Model file for the job. Use its own axes, mm. A direction names the side the tool comes from. Coordinates: 2 decimals unless noted, no trailing zeros. Write each loop counter-clockwise with the first axis right and the second up, starting at its lowest first coordinate (ties: lowest second). Pieces come first, ordered by that corner, then holes. Notation, with made-up numbers: (-27, 42) - (7, 42) arc R22 ccw to (7, 74) - close; hole circle Ø7 at (15.25, -40). An arc over 180 degrees is marked (long way). Put each result on its own line as item: value. Start each with the question number.
1. Saw through at B-B, the plane x = 0. Write the cut outline in (y, z) (1 decimal).
2. Drill centre lines: L1, parallel to Z at x = -21, y = -3 (3 decimals); L2, parallel to X at y = 2, z = -3; L3, parallel to X at y = 2, z = -9. Where is each one in solid material? Low to high. Write a range as from..to.
3. Saw through at D-D, the plane y = -2. Give the number of separate pieces and of enclosed holes in the cut face, plus the area to 3 significant figures.
4. Drop flat-ended pins along their axis: P1, Ø1, axis at y = -1, z = -24, coming from the +X side; P2, Ø4, axis at y = 1.5, z = -6, coming from the +X side; P3, Ø8, axis at y = 12, z = -5, coming from the -X side. Give the stop position or say it passes through.
5. Which spindle directions (+Z, -Z, +X, -X, +Y, -Y) get a long thin tool onto all of the face, cutting with end or side? Do faces 1 (the face through (1.27, 0, -24)), 2 (the face through (0, 0, -25.4)), 3 (the face through (0, 0, -22.225)). Say none if no direction does.
6. Saw through at C-C, the plane z = -12.5. Write the cut outline in (x, y) (1 decimal).
7. Pull direction Y, two halves, no side cores. Call faces 4 (the face through (-2.3, -4.4, 0)), 5 (the face through (-1.27, 0, -24)), 6 (the face through (7.559, 5.796, -3.541)): released by +Y, released by -Y, zero draft, split by the parting line, or undercut.
```python
from build123d import *

# Parameters (mm, degrees)
CUT_EXTRUDE1_DEPTH = 26.4
CUT_EXTRUDE2_DEPTH = 22.225
FILLET1_R          = 2.54


with BuildPart() as part:
    # Sketch1 → Revolve1 (revolve)
    with BuildSketch(Plane(origin=(0, 0, 0), x_dir=(1, 0, 0), z_dir=(0, 1, 0))):
        Polygon((0, 0), (-9.525, 0), (-9.525, 9.525), (-25.4, 9.525), (-25.4, 25.4), (0, 25.4), align=None)
    revolve(axis=Axis((0, 0, -87.406759955), (0, 0, 1)))

    # Sketch2 → Cut-Extrude1 (cut, through all)
    with BuildSketch(Plane(origin=(0, 0, -25.4), x_dir=(-1, 0, 0), z_dir=(0, 0, -1))):
        with BuildLine():
            Line((-1.27, -4.590044254), (-1.27, 4.590044254))
            ThreePointArc((-1.27, 4.590044254), (-4.7625, 0), (-1.27, -4.590044254))
        make_face()
        with BuildLine():
            ThreePointArc((4.7625, 0), (3.790104303, 2.883836962), (1.27, 4.590044254))
            Line((1.27, 4.590044254), (1.27, -4.590044254))
            ThreePointArc((1.27, -4.590044254), (3.790104303, -2.883836962), (4.7625, 0))
        make_face()
    extrude(amount=-CUT_EXTRUDE1_DEPTH, mode=Mode.SUBTRACT)

    # Sketch3 → Cut-Extrude2 (cut)
    with BuildSketch(Plane.XY):
        with BuildLine():
            ThreePointArc((1.27, 4.590044254), (0, 4.7625), (-1.27, 4.590044254))
            Line((-1.27, 4.590044254), (-1.27, -4.590044254))
            ThreePointArc((-1.27, -4.590044254), (0, -4.7625), (1.27, -4.590044254))
            Line((1.27, -4.590044254), (1.27, 4.590044254))
        make_face()
    extrude(amount=-CUT_EXTRUDE2_DEPTH, mode=Mode.SUBTRACT)

    # Fillet1
    fillet1_edges = [part.edges().sort_by_distance(p)[0] for p in [
        (9.525, 0, -9.525),
    ]]
    fillet(fillet1_edges, radius=FILLET1_R)


solid = part.part
```
Final values:
1. outline: (-25.4, -25.4) - (25.4, -25.4) - (25.4, -9.5) - (12.1, -9.5) arc R2.5 cw to (9.5, -7) - (9.5, 0) - (4.8, 0) - (4.8, -22.2) - (-4.8, -22.2) - (-4.8, 0) - (-9.5, 0) - (-9.5, -7) arc R2.5 cw to (-12.1, -9.5) - (-25.4, -9.5) - close
2. L1: z = -25.4..-9.525
2. L2: x = -9.31..-4.32, 4.32..9.31
2. L3: x = -10.33..-4.32, 4.32..10.33
3. separate pieces: 3
3. enclosed holes: 0
3. area: 773 mm²
4. P1: stops at x = 25.4
4. P2: stops at x = 9.66
4. P3: stops at x = -5.17
5. face 1: +Z, -Z
5. face 2: -Z, +X, -X, +Y, -Y
5. face 3: +Z
6. outline: circle Ø50.8 at (0, 0); hole circle Ø9.5 at (0, 0)
7. face 4: zero draft
7. face 5: undercut
7. face 6: split by the parting line
